Geometry: see drawing. Coordinates: mm, zero at the bounding-box minimum. A direction names the side the tool comes from. Round coordinates to 2 decimals unless told otherwise and drop trailing zeros. Write each loop counter-clockwise with the first axis right and the second up, starting at its lowest first coordinate (ties: lowest second). Pieces come first, ordered by that corner, then holes. Notation, with made-up numbers: M 84.25,-3.75 L 89.25,-3.75 A33 cw 89.25,27.25 Z; hole C 80.5,28.25 d7. An arc over 180 degrees is marked long. Use a Markdown table: item, result.
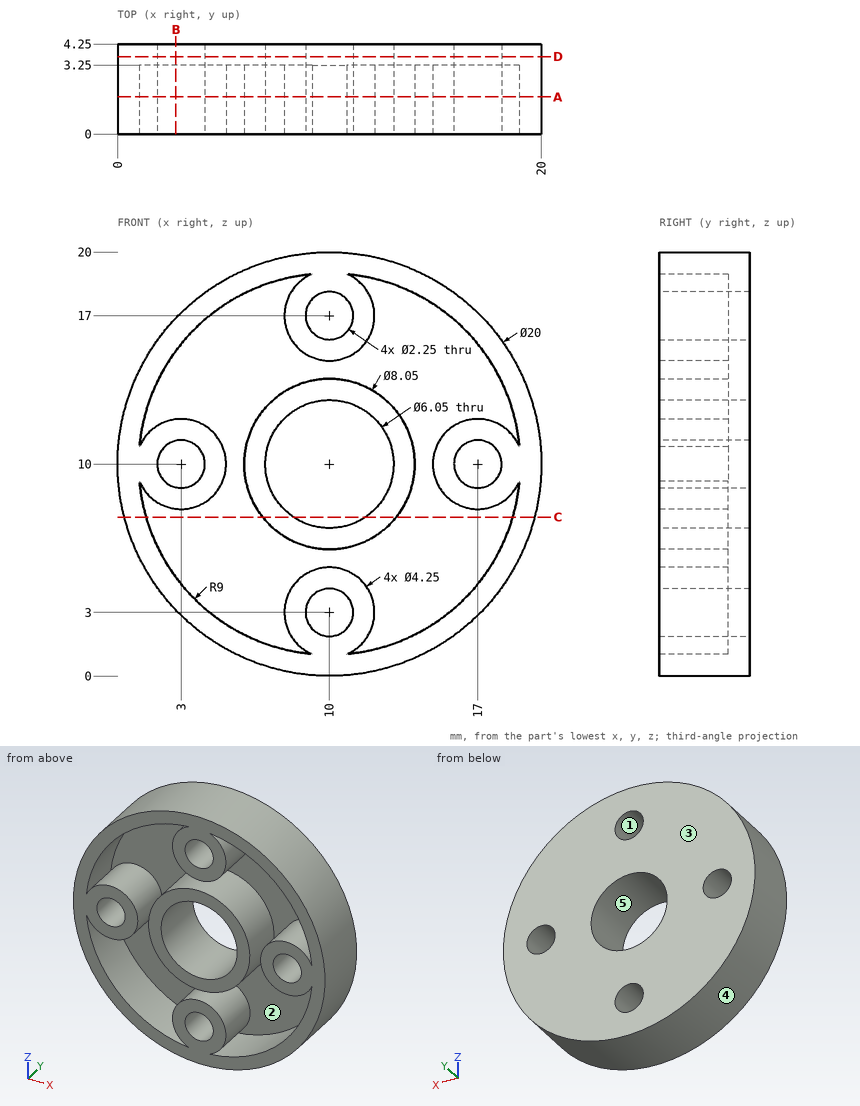
Q1. Line query: L1, parallel to X at y = 3.5, z = 10.25; L2, parallel to X at y = 1, z = 7.5; L3, parallel to Z at x = 18.25, y = 3.2. Output: solid intervals per line, ascending.
Results are:
| item | result |
|---|---|
| L1 | 0 to 1.9, 4.1 to 6.99, 13.01 to 15.9, 18.1 to 20 |
| L2 | 0.32 to 1.35, 6.85 to 8.3, 11.7 to 13.15, 18.65 to 19.68 |
| L3 | 4.35 to 6.4, 8.28 to 11.72, 13.6 to 15.65 |
Q2. Section B-B on x = 2.75. Return loops of the section in (y, z), plus the area to 3 significant figures.
Results are:
| item | result |
|---|---|
| outline | M 0,3.11 L 4.25,3.11 L 4.25,8.9 L 0,8.9 L 0,7.89 L 3.25,7.89 L 3.25,4.67 L 0,4.67 Z; M 0,11.1 L 4.25,11.1 L 4.25,16.89 L 0,16.89 L 0,15.33 L 3.25,15.33 L 3.25,12.11 L 0,12.11 Z |
| area | 28.3 mm^2 |
Q3. Section D-D on y = 3.65. Return loops of the section in (x, z) (3 decimals).
Results are:
| item | result |
|---|---|
| outline | C 10,10 d20; hole C 3,10 d2.25; hole C 10,10 d6.05; hole C 10,3 d2.25; hole C 10,17 d2.25; hole C 17,10 d2.25 |
Q4. Reachability of the marked faces 1 and 2 from +Z, -Z, +X, -X, +Y, -Y: full face, straight path, thin tool, end or side. Return the list, or none.
Results are:
| item | result |
|---|---|
| face 1 | +Y, -Y |
| face 2 | -Y |
Q5. Section A-A on y = 1.75. Return loops of the section in (x, z) (3 decimals), plus the area to 3 significant figures.
Results are:
| item | result |
|---|---|
| outline | C 10,10 d20; C 10,10 d8.05; hole M 1.037,9.187 A9 ccw 9.187,1.037 A2.125 cw long 10.813,1.037 A9 ccw 18.963,9.187 A2.125 cw long 18.963,10.813 A9 ccw 10.813,18.963 A2.125 cw long 9.187,18.963 A9 ccw 1.037,10.813 A2.125 cw long Z; hole C 3,10 d2.25; hole C 10,10 d6.05; hole C 10,3 d2.25; hole C 10,17 d2.25; hole C 17,10 d2.25 |
| area | 122 mm^2 |
Q6. First-contact query: pin 1 Ø1.5 at (x, y) = (15.5, 1.5) entering from -Z; pin 2 Ø1 at (x, y) = (7, 1.5) entering from +Z. Flat tips, straight axial feed; report the tip coordinate or a pass-through.
Results are:
| item | result |
|---|---|
| pin 1 | z = 1.2 |
| pin 2 | z = 19.68 |
Q7. Mould query, pull axis Z, two halves, no side actions, for the marked faces 3, 4 and 5. Classes: +Z half, -Z half, draft (parallel to the pull), parting line (faces both ways), or undercut.
Results are:
| item | result |
|---|---|
| face 3 | draft |
| face 4 | parting line |
| face 5 | undercut |
Q8. Section C-C on z = 7.5. Return loops of the section in (x, y), plus the area to 3 significant figures.
Results are:
| item | result |
|---|---|
| outline | M 0.32,0 L 1.35,0 L 1.35,3.25 L 6.85,3.25 L 6.85,0 L 8.3,0 L 8.3,4.25 L 0.32,4.25 Z; M 11.7,0 L 13.15,0 L 13.15,3.25 L 18.65,3.25 L 18.65,0 L 19.68,0 L 19.68,4.25 L 11.7,4.25 Z |
| area | 32.1 mm^2 |
